The model under review builds one solid part; all positions refer to its coordinate system, in mm. A direction names the side the tool comes from. Give positions to 0.01 mm unless a question says otherwise; leave off trailing zeros. Order: outer loops, then holes, each group sorted by start corner. A loop starts at its lowest first (then second) coordinate and runs counter-clockwise, first axis right, second up.
```python
from build123d import *

# Parameters (mm, degrees)
CROQUIS1_W              = 952.5
CROQUIS1_H              = 257.175
CROQUIS1_W_2            = 895.35
CROQUIS1_H_2            = 200.025
CROQUIS1_W_3            = 1028.7
CROQUIS1_H_3            = 317.5
SALIENTE_EXTRUIR1_DEPTH = 50.8
CROQUIS6_W              = 895.35
CROQUIS6_H              = 200.025
CROQUIS6_W_2            = 984.25
CROQUIS6_H_2            = 288.925
CORTAR_EXTRUIR6_DEPTH   = 47.625
CROQUIS1_4_W            = 895.35
CROQUIS1_4_H            = 200.025
CORTAR_EXTRUIR1_DEPTH   = 51.8
CROQUIS7_W              = 952.5
CROQUIS7_H              = 257.175
CORTAR_EXTRUIR7_DEPTH   = 51.8


with BuildPart() as part:
    # Croquis1 → Saliente-Extruir1 (new body)
    with BuildSketch(Plane(origin=(0, 0, 0), x_dir=(1, 0, 0), z_dir=(0, 1, 0))):
        Rectangle(CROQUIS1_W, CROQUIS1_H)
        Rectangle(CROQUIS1_W_2, CROQUIS1_H_2, mode=Mode.SUBTRACT)
        Rectangle(CROQUIS1_W_3, CROQUIS1_H_3)
        Rectangle(CROQUIS1_W, CROQUIS1_H, mode=Mode.SUBTRACT)
        Rectangle(CROQUIS1_W_2, CROQUIS1_H_2)
    extrude(amount=SALIENTE_EXTRUIR1_DEPTH)

    # Croquis6 → Cortar-Extruir6 (cut)
    with BuildSketch(Plane(origin=(0, 0, 0), x_dir=(-1, 0, 0), z_dir=(0, -1, 0))):
        Rectangle(CROQUIS6_W, CROQUIS6_H)
        Rectangle(CROQUIS6_W_2, CROQUIS6_H_2)
        Rectangle(CROQUIS6_W, CROQUIS6_H, mode=Mode.SUBTRACT)
    extrude(amount=-CORTAR_EXTRUIR6_DEPTH, mode=Mode.SUBTRACT)

    # Croquis1_4 → Cortar-Extruir1 (cut, through all)
    with BuildSketch(Plane(origin=(0, 0, 0), x_dir=(1, 0, 0), z_dir=(0, 1, 0))):
        Rectangle(CROQUIS1_4_W, CROQUIS1_4_H)
    extrude(amount=CORTAR_EXTRUIR1_DEPTH, mode=Mode.SUBTRACT)

    # Croquis7 → Cortar-Extruir7 (cut, through all)
    with BuildSketch(Plane(origin=(0, 50.8, 0), x_dir=(1, 0, 0), z_dir=(0, 1, 0))):
        Rectangle(CROQUIS7_W, CROQUIS7_H)
    extrude(amount=-CORTAR_EXTRUIR7_DEPTH, mode=Mode.SUBTRACT)


solid = part.part
```
Item 1: Take a section at B-B (z = -98). Give the boundary of the cut face in (x, y) (3 decimals).
Values found:
outline: (-514.35, 0) - (-492.125, 0) - (-492.125, 47.625) - (-476.25, 47.625) - (-476.25, 50.8) - (-514.35, 50.8) - close; (476.25, 47.625) - (492.125, 47.625) - (492.125, 0) - (514.35, 0) - (514.35, 50.8) - (476.25, 50.8) - close
Item 2: For line 1 (Z direction, x = 169.5, y = 28.5); line 2 (X direction, y = 11, z = -2.5) (3 decimals); line 3 (Y direction, x = -9, z = 135.5) (3 decimals), list the stretches that pass through material, from the lowest coordinate up.
Values found:
line 1: z = -158.75 to -144.46, 144.46 to 158.75
line 2: x = -514.35 to -492.125, 492.125 to 514.35
line 3: y = 47.625 to 50.8
Item 3: Draft analysis for pull direction Z (two halves, no side actions). For faces 3 (the flat face through (7, 23, 144.462)), 4 (the flat face through (-7, 25, -158.75)), 5 (the flat face through (-41, 0, 152)), state which applies: released by +Z, released by -Z, zero draft, split by the parting line, or undercut.
Values found:
face 3: undercut
face 4: released by -Z
face 5: zero draft
Item 4: For faces 1 (the flat face through (-492.125, 23, 2)), 2 (the flat face through (514.35, 25, 2)), list the 3-axis set-ups (+Z, -Z, +X, -X, +Y, -Y) from which the entire face can be reached by the end or side of a thin tool; tool diameter is ignored.
Values found:
face 1: -Y
face 2: +Z, -Z, +X, +Y, -Y
